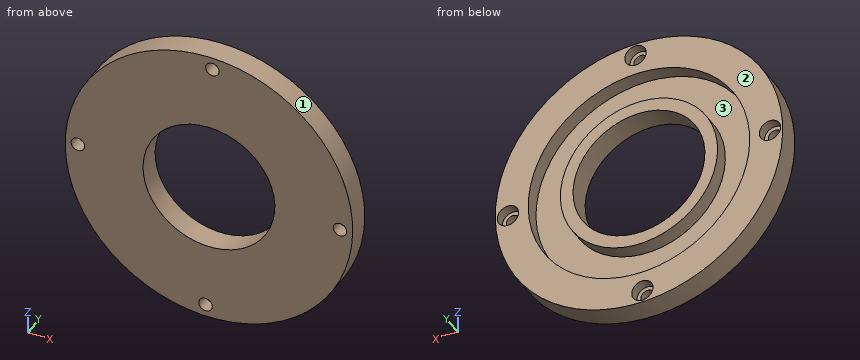
from build123d import *

# Parameters (mm, degrees)
SKETCH1_R           = 42.5
SKETCH1_R_2         = 19.5
BOSS_EXTRUDE1_DEPTH = 7
SKETCH2_R           = 32.75
SKETCH2_R_2         = 23.25
CUT_EXTRUDE1_DEPTH  = 4.5
SKETCH3_R           = 2
CUT_EXTRUDE2_DEPTH  = 61.510329697
SKETCH4_R           = 3.15
SKETCH4_R_2         = 2
CUT_EXTRUDE3_DEPTH  = 3


with BuildPart() as part:
    # Sketch1 → Boss-Extrude1 (new body)
    with BuildSketch(Plane(origin=(0, 0, 0), x_dir=(1, 0, 0), z_dir=(0, 1, 0))):
        with Locations(Location((0, 0, 0), (0, 0, 270))):
            Circle(SKETCH1_R)
        with Locations(Location((0, 0, 0), (0, 0, 270))):
            Circle(SKETCH1_R_2, mode=Mode.SUBTRACT)
    extrude(amount=BOSS_EXTRUDE1_DEPTH)

    # Sketch2 → Cut-Extrude1 (cut)
    with BuildSketch(Plane(origin=(0, 7, 0), x_dir=(1, 0, 0), z_dir=(0, 1, 0))):
        with Locations(Location((0, 0, 0), (0, 0, 270))):
            Circle(SKETCH2_R)
        with Locations(Location((0, 0, 0), (0, 0, 270))):
            Circle(SKETCH2_R_2, mode=Mode.SUBTRACT)
    extrude(amount=-CUT_EXTRUDE1_DEPTH, mode=Mode.SUBTRACT)

    # Sketch3 → Cut-Extrude2 (cut, through all)
    with BuildSketch(Plane(origin=(0, 7, 0), x_dir=(1, 0, 0), z_dir=(0, 1, 0))):
        with Locations(Location((-38.75, -1.015406046, 0), (0, 0, 270))):
            Circle(SKETCH3_R)
        with Locations(Location((-1.015406046, 38.75, 0), (0, 0, 270))):
            Circle(SKETCH3_R)
        with Locations(Location((38.75, 1.015406046, 0), (0, 0, 270))):
            Circle(SKETCH3_R)
        with Locations(Location((1.015406046, -38.75, 0), (0, 0, 270))):
            Circle(SKETCH3_R)
    extrude(amount=-CUT_EXTRUDE2_DEPTH, mode=Mode.SUBTRACT)

    # Sketch4 → Cut-Extrude3 (cut)
    # profile 1 of 4: a face of its own
    with BuildSketch(Plane(origin=(0, 7, 0), x_dir=(1, 0, 0), z_dir=(0, 1, 0))):
        with Locations(Location((-1.015406046, 38.75, 0), (0, 0, 270))):
            Circle(SKETCH4_R)
        with Locations(Location((-1.015406046, 38.75, 0), (0, 0, 270))):
            Circle(SKETCH4_R_2, mode=Mode.SUBTRACT)
    # profile 2 of 4: a face of its own
    with BuildSketch(Plane(origin=(0, 7, 0), x_dir=(1, 0, 0), z_dir=(0, 1, 0))):
        with Locations(Location((38.75, 1.015406046, 0), (0, 0, 270))):
            Circle(SKETCH4_R)
    # profile 3 of 4: a face of its own
    with BuildSketch(Plane(origin=(0, 7, 0), x_dir=(1, 0, 0), z_dir=(0, 1, 0))):
        with Locations(Location((1.015406046, -38.75, 0), (0, 0, 270))):
            Circle(SKETCH4_R)
    # profile 4 of 4: a face of its own
    with BuildSketch(Plane(origin=(0, 7, 0), x_dir=(1, 0, 0), z_dir=(0, 1, 0))):
        with Locations(Location((-38.75, -1.015406046, 0), (0, 0, 270))):
            Circle(SKETCH4_R)
    extrude(amount=-CUT_EXTRUDE3_DEPTH, mode=Mode.SUBTRACT)


solid = part.part
Read the model definition and answer for the solid it produces. Units are mm, in the model's axes. Face numbers are marked on the shaded views. Give positions to 0.01 mm unless a question says otherwise; leave off trailing zeros. Write each loop counter-clockwise with the first axis right and the second up, starting at its lowest first coordinate (ties: lowest second). Pieces come first, ordered by that corner, then holes. Notation, with made-up numbers: (7, -9) - (59, -9) arc R25 ccw to (59, 3) - close; hole circle Ø7 at (71, -37). An arc over 180 degrees is marked (long way). Answer in a Markdown table with one row per item. Add a question column.
Item 1: Section B-B, the plane x = 6 is taken. Write down the section's boundary in (y, z).
Item 2: Find the intervals of material crossed by L1, parallel to Z at x = 1, y = 5; L2, parallel to X at y = 4, z = 9; L3, parallel to Z at x = 21, y = 5.75, in increasing order.
Item 3: Section C-C, the plane z = 0 is taken. Count the separate pieces of the cut face and the enclosed holes in it, and give its area (3 significant figures).
Item 4: Section A-A, the plane y = 5.5 is taken. Write down the section's boundary in (x, z).
Item 5: Section D-D, the plane z = -18.5 is taken. Write down the section's boundary in (x, y).
Item 6: Determine the mould class of the marked faces 1, 2 and 3 for opening direction Z: pulls with the +Z half, pulls with the -Z half, needs draft (parallel to the pull), parting line crosses it, or undercut.
Item 7: Flat-ended cylindrical pins translate along their axes: P1, Ø1, axis at y = 6, z = 15, coming from the +X side; P2, Ø5, axis at x = 38.75, z = -1.02, coming from the +Y side; P3, Ø2, axis at x = -22.5, y = 3.5, coming from the -Z side. Find the tip coordinate at first contact, or state that the pin passes through.
Recorded:
| question | item | result |
|---|---|---|
| 1 | outline | (0, -42.07) - (7, -42.07) - (7, -32.2) - (2.5, -32.2) - (2.5, -22.46) - (7, -22.46) - (7, -18.55) - (0, -18.55) - close; (0, 18.55) - (7, 18.55) - (7, 22.46) - (2.5, 22.46) - (2.5, 32.2) - (7, 32.2) - (7, 42.07) - (0, 42.07) - close |
| 2 | L1 | z = -42.49 to -41.17, -36.33 to -32.73, -23.23 to -19.47, 19.47 to 23.23, 32.73 to 35.6, 41.9 to 42.49 |
| 2 | L2 | x = -41.54 to -31.49, -21.44 to -17.3, 17.3 to 21.44, 31.49 to 41.54 |
| 2 | L3 | z = -36.95 to -25.13, -9.98 to 9.98, 25.13 to 36.95 |
| 3 | separate pieces | 4 |
| 3 | enclosed holes | 0 |
| 3 | area | 173 mm2 |
| 4 | outline | circle Ø85 at (0, 0); circle Ø46.5 at (0, 0); hole circle Ø6.3 at (-38.75, 1.02); hole circle Ø65.5 at (0, 0); hole circle Ø39 at (0, 0); hole circle Ø6.3 at (-1.02, -38.75); hole circle Ø6.3 at (1.02, 38.75); hole circle Ø6.3 at (38.75, -1.02) |
| 5 | outline | (-38.26, 0) - (-6.16, 0) - (-6.16, 7) - (-14.08, 7) - (-14.08, 2.5) - (-27.02, 2.5) - (-27.02, 7) - (-38.26, 7) - close; (6.16, 0) - (38.26, 0) - (38.26, 7) - (27.02, 7) - (27.02, 2.5) - (14.08, 2.5) - (14.08, 7) - (6.16, 7) - close |
| 6 | face 1 | parting line crosses it |
| 6 | face 2 | needs draft |
| 6 | face 3 | undercut |
| 7 | P1 | stops at x = 39.95 |
| 7 | P2 | stops at y = 4 |
| 7 | P3 | stops at z = -36.66 |
